from build123d import *

# Parameters (mm, degrees)
F1_DEPTH = 46.9760447741
F3_DEPTH = 48.9080855623
F6_DEPTH = 47.6816631854


with BuildPart() as f1:
    # F0 (on Top) → F1 (new body)
    with BuildSketch(Plane.XY):
        with BuildLine():
            ThreePointArc((-71.2393962349, 32.9179256613), (53.631854808, -144.2703545516), (215.4174560814, 0))
            ThreePointArc((215.4174560814, 0), (212.4239330052, 29.333743716), (203.5667803118, 57.4581200997))
            ThreePointArc((203.5667803118, 57.4581200997), (180.7556781079, 94.1574324953), (148.1557889137, 122.5199630346))
            ThreePointArc((148.1557889137, 122.5199630346), (71.7340942101, 145.2103590343), (-5.1502163644, 124.140658527))
            ThreePointArc((-5.1502163644, 124.140658527), (-47.4003805504, 85.1985600864), (-71.2393962349, 32.9179256613))
        make_face()
        with BuildLine():
            ThreePointArc((148.1557889137, 122.5199630346), (180.7556781079, 94.1574324953), (203.5667803118, 57.4581200997))
            ThreePointArc((203.5667803118, 57.4581200997), (236.1595707678, 139.7134864477), (183.5359483957, 210.840061307))
            ThreePointArc((183.5359483957, 210.840061307), (159.5565215905, 169.199462517), (148.1557889137, 122.5199630346))
        make_face()
        with BuildLine():
            ThreePointArc((-69.5170983672, 185.6363117695), (-98.925732723, 109.5990660233), (-71.2393962349, 32.9179256613))
            ThreePointArc((-71.2393962349, 32.9179256613), (-47.4003805504, 85.1985600864), (-5.1502163644, 124.140658527))
            ThreePointArc((-5.1502163644, 124.140658527), (-34.3996197413, 157.9595128325), (-69.5170983672, 185.6363117695))
        make_face()
    extrude(amount=-F1_DEPTH)

    # F2 (on face) → F3 (join)
    with BuildSketch(Plane.XY):
        with BuildLine():
            ThreePointArc((44.9946392241, 143.0144957499), (71.2893502257, 145.2143795795), (97.5480618405, 142.6198892915))
            ThreePointArc((97.5480618405, 142.6198892915), (71.7551928662, 207.2549889957), (44.9946392241, 143.0144957499))
        make_face()
    extrude(amount=-F3_DEPTH)

    # F5 (on face) → F6 (join)
    with BuildSketch(Plane.XY):
        with BuildLine():
            ThreePointArc((-75.0189256599, -0.404913858), (-74.9976500667, 2.5184711417), (-74.917529707, 5.4408354645))
            Line((-74.917529707, 5.4408354645), (-105.7080030441, 24.6027484536))
            Line((-105.7080030441, 24.6027484536), (-108.3586743244, 20.3434960801))
            Line((-108.3586743244, 20.3434960801), (-75.0189256599, -0.404913858))
        make_face()
        with BuildLine():
            ThreePointArc((-69.9400027769, -38.0719006061), (-70.6055307061, -35.5315897531), (-71.2250142357, -32.9796597362))
            Line((-71.2250142357, -32.9796597362), (-130.4813623428, -32.9796597362))
            Line((-130.4813623428, -32.9796597362), (-130.4813623428, -38.0719006062))
            Line((-130.4813623428, -38.0719006062), (-69.9400027769, -38.0719006062))
        make_face()
        with BuildLine():
            ThreePointArc((-55.7230830607, -72.3328295314), (-57.207340031, -69.6852480865), (-58.6359381198, -67.0072238594))
            Line((-58.6359381198, -67.0072238594), (-87.6557826996, -86.5481868386))
            Line((-87.6557826996, -86.5481868386), (-84.2797279511, -91.561889807))
            Line((-84.2797279511, -91.561889807), (-55.7230830607, -72.3328295314))
        make_face()
        with BuildLine():
            ThreePointArc((215.2245101702, -7.483407855), (215.0646070932, -10.1171082931), (214.8568793088, -12.747468755))
            Line((214.8568793088, -12.747468755), (285.2909564972, -12.4354660511))
            Line((285.2909564972, -12.4354660511), (285.3941321373, -7.483407855))
            Line((285.3941321373, -7.483407855), (215.2245101702, -7.483407855))
        make_face()
        with BuildLine():
            ThreePointArc((210.7247036656, -36.618666769), (210.1115019764, -38.8959118449), (209.4613997229, -41.1628985028))
            Line((209.4613997229, -41.1628985028), (261.3650764015, -49.1495164643))
            Line((261.3650764015, -49.1495164643), (262.0773613453, -44.5204973221))
            Line((262.0773613453, -44.5204973221), (210.7247036656, -36.618666769))
        make_face()
        with BuildLine():
            Line((267.1763300896, 32.936360687), (213.9242377293, 20.7715208216))
            ThreePointArc((213.9242377293, 20.7715208216), (214.1894129137, 18.8457161569), (214.4287850178, 16.9165343406))
            Line((214.4287850178, 16.9165343406), (268.0576479304, 29.0783551911))
            Line((268.0576479304, 29.0783551911), (267.1763300896, 32.936360687))
        make_face()
    extrude(amount=-F6_DEPTH)


solid = f1.part
Source: CAD feature listing. Evaluate the final solid. Frame: model axes, mm. A direction names the side the tool comes from. Coordinates: 2 decimals unless noted, no trailing zeros. Loops run counter-clockwise (first coordinate to the right, second up) from the corner with the lowest first, then second, coordinate; pieces in that order, holes last. Notation, with made-up numbers: (57.5, 46.5) - (113.5, 46.5) arc R25 ccw to (113.5, 60.5) - close; hole circle Ø3 at (41.5, 28). An arc over 180 degrees is marked (long way). One line per question, with ' | ' between items.
1) Section B-B, the plane x = -93. Return loops of the section in (y, z), then the cut area to 3 significant figures.
Report:
outline: (-38.07, -47.68) - (-32.98, -47.68) - (-32.98, 0) - (-38.07, 0) - close; (10.79, -47.68) - (16.69, -47.68) - (16.69, 0) - (10.79, 0) - close; (71.6, -46.98) - (144.98, -46.98) - (144.98, 0) - (71.6, 0) - close | area: 3,970 mm²
2) Pull-direction query (X, two-part tool) for faces 1 (the face through (-72, -80, -47.682)), 2 (the face through (124.16, 134.82, -23.16)), 3 (the face through (-98.907, 110.765, -23.159)); classes: released by +X, released by -X, zero draft, split by the parting line, or undercut.
Report:
face 1: zero draft | face 2: undercut | face 3: released by -X
3) Section C-C, the plane x = 53. Return loops of the section in (y, z), then the cut area to 3 significant figures.
Report:
outline: (-144.2, -46.98) - (144.2, -46.98) - (144.2, -48.91) - (202.4, -48.91) - (202.4, 0) - (-144.2, 0) - close | area: 16,400 mm²
4) Set-up query: faces 4 (the face through (-90.1, 14.89, -23.51)), 5 (the face through (-100, -32.98, -24)), 6 (the face through (-70.2, -82.08, -23.51)). Return all of +Z, -Z, +X, -X, +Y, -Y with unobstructed straight access to the full face (end or side cutting, diameter ignored); none if empty.
Report:
face 4: +Z, -Z | face 5: +Z, -Z, -X | face 6: +Z, -Z, -Y
5) Line query: line 1 along Y through (x, z) = (-83, -26); line 2 along X through (y, z) = (-6.5, -43.5); line 3 along X through (y, z) = (125, -18). Output: solid intervals per line, ascending.
Report:
line 1: y = -90.7 to -83.41, -38.07 to -32.98, 4.56 to 10.47, 49.5 to 167.07 | line 2: x = -74.87 to 215.27 | line 3: x = -97.73 to -5.76, -3.72 to 144.11, 148.42 to 236.88
6) Section D-D, the plane y = -109. Return loops of the section in (x, z).
Report:
outline: (-25.76, -46.98) - (166.15, -46.98) - (166.15, 0) - (-25.76, 0) - close
7) First-contact query: P1, Ø5, axis at y = 12, z = -18.5, coming from the +X side; P2, Ø14.5, axis at x = -114.5, z = -25, coming from the -Y side; P3, Ø8, axis at x = 92.5, z = -20.5, coming from the +Y side; P4, Ø1.5, axis at x = -17, y = -55, coming from the +Z side. Flat tips, straight axial feed; report the tip coordinate or a pass-through.
Report:
P1: stops at x = 215.11 | P2: stops at y = -38.07 | P3: stops at y = 203.18 | P4: stops at z = 0
